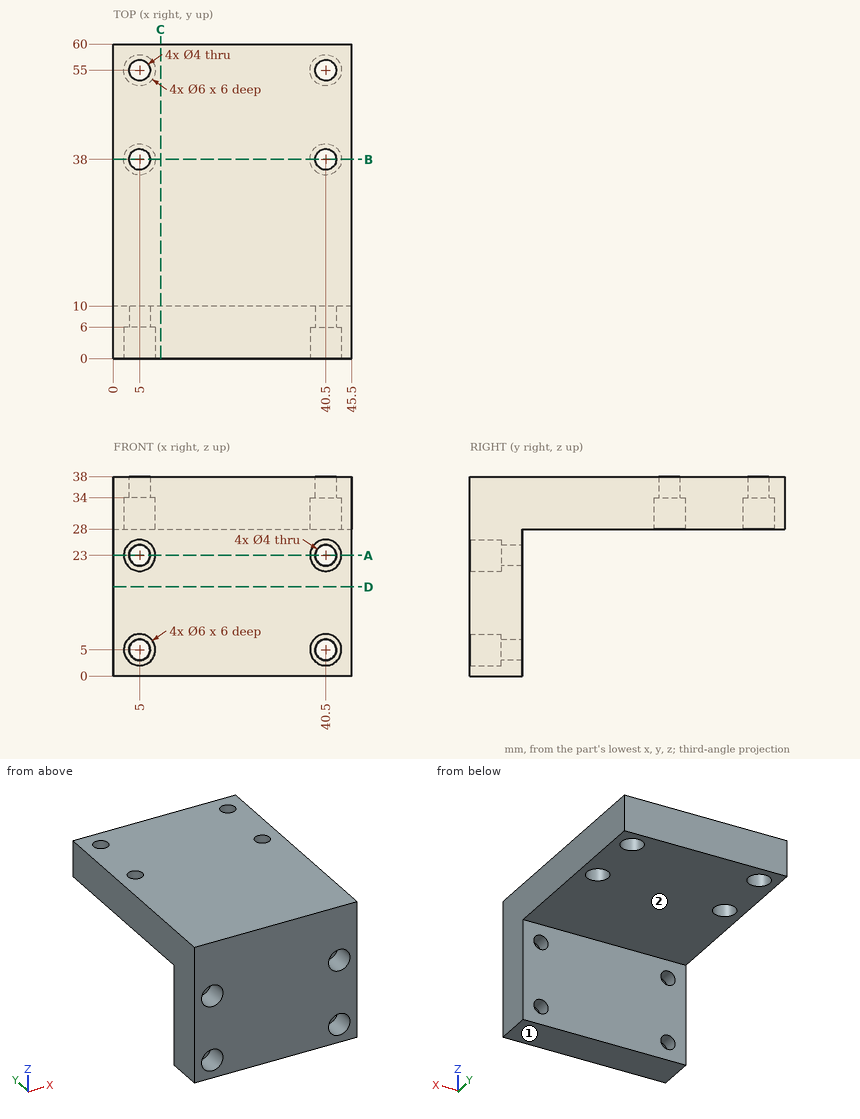
Check sheet for the drawn part. Datum: minimum x, y, z corner. Units: mm. A direction names the side the tool comes from. Round coordinates to 2 decimals unless told otherwise and drop trailing zeros. Write each loop counter-clockwise with the first axis right and the second up, starting at its lowest first coordinate (ties: lowest second). Pieces come first, ordered by that corner, then holes. Notation, with made-up numbers: (83.25, 57.5) - (142.25, 57.5) arc R28 ccw to (142.25, 85.5) - close; hole circle Ø11 at (72, 29.25). An arc over 180 degrees is marked (long way). Return JSON: item names as keys, results as strings.
Q1. Cross-section at D-D (z = 17). Record the boundary of the cut face in (x, y).
Returned:
{"outline": "(0, 0) - (45.5, 0) - (45.5, 10) - (0, 10) - close"}
Q2. Access from +Z, -Z, +X, -X, +Y, -Y to the whole of each face (thin tool, end or side, straight path). Record for the marked faces 1 and 2.
Returned:
{"face 1": "-Z, +X, -X, +Y, -Y", "face 2": "-Z, +X, -X, +Y"}
Q3. Depth check by flat-ended pin: P1, Ø3, axis at x = 40.5, z = 23, coming from the -Y side; P2, Ø3, axis at x = 22.5, y = 42.5, coming from the -Z side; P3, Ø3, axis at x = 4.5, z = 6, coming from the -Y side; P4, Ø6.5, axis at x = 5, z = 5, coming from the +Y side. Enter the tip coordinate at first touch or a pass-through.
Returned:
{"P1": "passes through", "P2": "stops at z = 28", "P3": "stops at y = 6", "P4": "stops at y = 10"}
Q4. Cross-section at A-A (z = 23). Record the boundary of the cut face in (x, y), then the cut area to 3 significant figures.
Returned:
{"outline": "(0, 0) - (2, 0) - (2, 6) - (3, 6) - (3, 10) - (0, 10) - close; (7, 6) - (8, 6) - (8, 0) - (37.5, 0) - (37.5, 6) - (38.5, 6) - (38.5, 10) - (7, 10) - close; (42.5, 6) - (43.5, 6) - (43.5, 0) - (45.5, 0) - (45.5, 10) - (42.5, 10) - close", "area": "351 mm²"}
Q5. Cross-section at C-C (x = 9). Record the boundary of the cut face in (y, z), then the cut area to 3 significant figures.
Returned:
{"outline": "(0, 0) - (10, 0) - (10, 28) - (60, 28) - (60, 38) - (0, 38) - close", "area": "880 mm²"}
Q6. Scan lines: L1, parallel to X at y = 9, z = 5; L2, parallel to Z at x = 5, y = 8; L3, parallel to Y at x = 40.5, z = 35. Record each from-to range of solid material in increasing order. Write a range as from..to.
Returned:
{"L1": "x = 0..3, 7..38.5, 42.5..45.5", "L2": "z = 0..3, 7..21, 25..38", "L3": "y = 0..36, 40..53, 57..60"}
Q7. Cross-section at B-B (y = 38). Record the boundary of the cut face in (x, z).
Returned:
{"outline": "(0, 28) - (2, 28) - (2, 34) - (3, 34) - (3, 38) - (0, 38) - close; (7, 34) - (8, 34) - (8, 28) - (37.5, 28) - (37.5, 34) - (38.5, 34) - (38.5, 38) - (7, 38) - close; (42.5, 34) - (43.5, 34) - (43.5, 28) - (45.5, 28) - (45.5, 38) - (42.5, 38) - close"}
